from build123d import *

# Parameters (mm, degrees)
SKETCH1_W               = 100
SKETCH1_H               = 64
BOSS_EXTRUDE1_DEPTH     = 22
CUT_EXTRUDE1_DEPTH      = 108.275346655
CUT_EXTRUDE1_DEPTH_BACK = 108.275346655
SKETCH4_W               = 15
SKETCH4_H               = 64
BOSS_EXTRUDE2_DEPTH     = 53
CHAMFER1_START          = 64.346717088
CHAMFER1_OUTLINE_W      = 15
CHAMFER1_OUTLINE_H      = 25
CHAMFER1_DEPTH          = 12.653282912
CHAMFER2_START          = 64.346717088
CHAMFER2_OUTLINE_W      = 15
CHAMFER2_OUTLINE_H      = 25
CHAMFER2_DEPTH          = 12.653282912
RIB1_REACH              = 97.65
SKETCH5_WALL_W          = 273.923387726
SKETCH5_WALL_H          = 12


with BuildPart() as part:
    # Sketch1 → Boss-Extrude1 (new body)
    with BuildSketch(Plane(origin=(0, 0, 0), x_dir=(1, 0, 0), z_dir=(0, 1, 0))):
        Rectangle(SKETCH1_W, SKETCH1_H)
    extrude(amount=BOSS_EXTRUDE1_DEPTH)

    # Sketch2 → Cut-Extrude1 (cut, two sides: drawn at the far end of the back side and taken through both)
    with BuildSketch(Plane(origin=(50, 0, 0), x_dir=(0, 0, -1), z_dir=(1, 0, 0)).offset(-CUT_EXTRUDE1_DEPTH_BACK)):
        Polygon((-43.110063235, -82.552699055), (4.551759787, 0), (11.479963017, 12), (-11.479963017, 12), (-4.551759787, 0), (43.110063235, -82.552699055), (43.110063235, 108.094593032), (-43.110063235, 108.094593032), align=None)
    extrude(amount=CUT_EXTRUDE1_DEPTH + CUT_EXTRUDE1_DEPTH_BACK, mode=Mode.SUBTRACT)

    # Sketch4 → Boss-Extrude2 (add)
    with BuildSketch(Plane(origin=(0, 22, 0), x_dir=(1, 0, 0), z_dir=(0, 1, 0))):
        with Locations((-42.5, 0)):
            Rectangle(SKETCH4_W, SKETCH4_H)
    extrude(amount=BOSS_EXTRUDE2_DEPTH)

    # Chamfer1: read off the stored shape, not the designer's step
    # Chamfer1 outline → Chamfer1 (cut)
    with BuildSketch(Plane(origin=(0, 0, 0), x_dir=(1, 0, 0), z_dir=(0, 0.7071067811865476, 0.7071067811865476)).offset(CHAMFER1_START)):
        with Locations((-42.5, 30.5)):
            Rectangle(CHAMFER1_OUTLINE_W, CHAMFER1_OUTLINE_H)
    extrude(amount=CHAMFER1_DEPTH, mode=Mode.SUBTRACT)

    # Chamfer2: read off the stored shape, not the designer's step
    # Chamfer2 outline → Chamfer2 (cut)
    with BuildSketch(Plane(origin=(0, 0, 0), x_dir=(1, 0, 0), z_dir=(0, 0.7071067811865476, -0.7071067811865476)).offset(CHAMFER2_START)):
        with Locations((-42.5, -30.5)):
            Rectangle(CHAMFER2_OUTLINE_W, CHAMFER2_OUTLINE_H)
    extrude(amount=CHAMFER2_DEPTH, mode=Mode.SUBTRACT)

    # Sketch5 wall → Rib1 (add, up to next)
    with BuildSketch(Plane(origin=(0, 42, 0), x_dir=(0.868243142124, -0.496138938357, 0), z_dir=(0.496138938357, 0.868243142124, 0)), mode=Mode.PRIVATE) as rib1_sk1:
        Rectangle(SKETCH5_WALL_W, SKETCH5_WALL_H)
    rib1_tool1 = extrude(rib1_sk1.sketch, amount=-RIB1_REACH, mode=Mode.PRIVATE) - part.part
    add(rib1_tool1.solids().sort_by_distance((0, 42, 0))[0])


solid = part.part
Can you work these out from the model? Positions are in its coordinate system, mm. A direction names the side the tool comes from. Coordinates: 2 decimals unless noted, no trailing zeros. Loops run counter-clockwise (first coordinate to the right, second up) from the corner with the lowest first, then second, coordinate; pieces in that order, holes last. Notation, with made-up numbers: (-16, 7.5) - (33, 7.5) arc R8 ccw to (33, 17.5) - close; hole circle Ø1 at (-26, 42.5). An arc over 180 degrees is marked (long way). Answer as a JSON object with one key per item and string values. Group by question number.
Item 1: If we section it at C-C (z = -9): List the corners of the cut face in (x, y) for me, plus the area to 3 significant figures.
Item 2: If we mould it in two halves opening along Z, with no side actions, what happens to faces 1 (the face through (7, 22, -8)), 2 (the face through (-13, 39, 6)), 3 (the face through (-1, 12, 0))? For each: released by +Z, released by -Z, zero draft, split by the parting line, or undercut.
Item 3: If we section it at D-D (y = 36): List the corners of the cut face in (x, z) for me.
Item 4: For pin 1 (1 mm diameter, centred on y = 63.5, z = 19, fed in from +X); pin 2 (2 mm diameter, centred on x = -1.5, z = 1, fed in from +Y), each with a flat end and sliding along its axis, tell me the tip position at first contact or that it passes through.
Item 5: If we section it at A-A (z = 2): List the corners of the cut face in (x, y) for me, plus the area to 4 significant figures.
Item 6: If I drill on L1, parallel to X at y = 59, z = -19; L2, parallel to Z at x = 27.5, y = 9; L3, parallel to Y at x = 45, z = 15, over which ranges is the centre line in solid material (lowest first)? Write a range as from..to.
Item 7: On a 3-axis mill with a long thin cutter (end or side, diameter ignored), from which of +Z, -Z, +X, -X, +Y, -Y can I reach the whole of each face in a straight line? I mean faces 4 (the face through (-35, 48, -7)), 5 (the face through (-0.7, 6.08, 8.06)), 6 (the face through (-1, 0, -18)), 7 (the face through (-13, 39, -6)), 8 (the face through (-43, 67, 24)). Say none if no direction works.
Item 8: If we section it at B-B (x = 10.5): List the corners of the cut face in (y, z) for me.
Returned:
{
 "1": {"outline": "(-50, 0) - (50, 0) - (50, 7.7) - (-50, 7.7) - close; (-50, 12) - (50, 12) - (50, 22) - (-35, 22) - (-35, 75) - (-50, 75) - close", "area": "2,570 mm²"},
 "2": {"face 1": "zero draft", "face 2": "released by +Z", "face 3": "undercut"},
 "3": {"outline": "(-50, -32) - (-35, -32) - (-35, -6) - (10.5, -6) - (10.5, 6) - (-35, 6) - (-35, 32) - (-50, 32) - close"},
 "4": {"pin 1": "stops at x = -35", "pin 2": "stops at y = 43.43"},
 "5": {"outline": "(-50, 12) - (50, 12) - (50, 22) - (35, 22) - (-35, 62) - (-35, 75) - (-50, 75) - close", "area": "3,195 mm²"},
 "6": {"L1": "x = -50..-35", "L2": "z = -32..-9.75, 9.75..32", "L3": "y = 0..22"},
 "7": {"face 4": "+X, +Y", "face 5": "+X, -X", "face 6": "+Z, -Z, +X, -X, -Y", "face 7": "-Z, +X, +Y", "face 8": "+Z, +X, -X, +Y"},
 "8": {"outline": "(0, -32) - (22, -32) - (22, -6) - (36, -6) - (36, 6) - (22, 6) - (22, 32) - (0, 32) - (0, 4.55) - (12, 11.48) - (12, -11.48) - (0, -4.55) - close"}
}
